from build123d import *

# Parameters (mm, degrees)
SKETCH1_W           = 114.24
SKETCH1_H           = 10
BOSS_EXTRUDE1_DEPTH = 10
SKETCH3_W           = 114.24
SKETCH3_H           = 10
BOSS_EXTRUDE2_DEPTH = 80
SKETCH4_R           = 4
CUT_EXTRUDE1_DEPTH  = 103.896522779


with BuildPart() as part:
    # Sketch1 → Boss-Extrude1 (new body)
    with BuildSketch(Plane.XY):
        Rectangle(SKETCH1_W, SKETCH1_H)
    extrude(amount=BOSS_EXTRUDE1_DEPTH)

    # Sketch3 → Boss-Extrude2 (add)
    with BuildSketch(Plane(origin=(0, 5, 0), x_dir=(1, 0, 0), z_dir=(0, 1, 0))):
        with Locations((0, -5)):
            Rectangle(SKETCH3_W, SKETCH3_H)
    extrude(amount=BOSS_EXTRUDE2_DEPTH)

    # Sketch4 → Cut-Extrude1 (cut, through all)
    with BuildSketch(Plane.XY.offset(10)):
        with Locations((24.87, 9.99)):
            Circle(SKETCH4_R)
    extrude(amount=-CUT_EXTRUDE1_DEPTH, mode=Mode.SUBTRACT)


solid = part.part
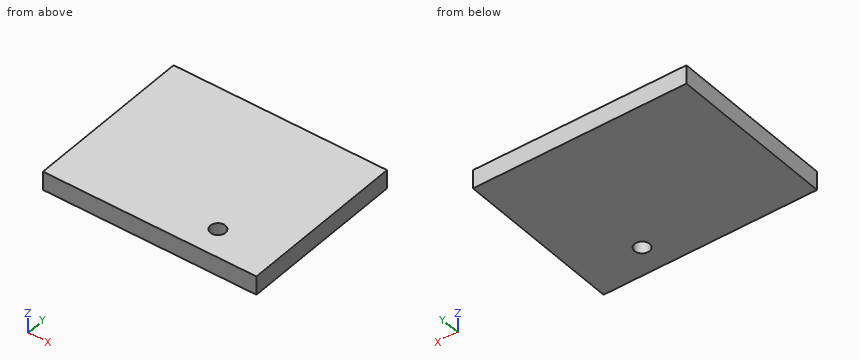
Here's how the part is built. I have some questions about the finished solid (model axes, mm). Round coordinates to 2 decimals unless told otherwise and drop trailing zeros. Write each loop counter-clockwise with the first axis right and the second up, starting at its lowest first coordinate (ties: lowest second). Pieces come first, ordered by that corner, then holes.
1. Suppose I cut it at A-A (y = 9.99). List the corners of the cut face in (x, z) for me.
2. Suppose I cut it at B-B (x = 24.87). List the corners of the cut face in (y, z) for me.
3. I need wall thicknesses on L1, parallel to Y at x = 24.87, z = 7.5; L2, parallel to X at y = 7, z = 0.5; L3, parallel to Y at x = 26, z = 9. Which ranges of each line are inside material? Lowest first, please.
Answer sheet:
1. outline: (-57.12, 0) - (20.87, 0) - (20.87, 10) - (-57.12, 10) - close; (28.87, 0) - (57.12, 0) - (57.12, 10) - (28.87, 10) - close
2. outline: (-5, 0) - (5.99, 0) - (5.99, 10) - (-5, 10) - close; (13.99, 0) - (85, 0) - (85, 10) - (13.99, 10) - close
3. L1: y = -5 to 5.99, 13.99 to 85
3. L2: x = -57.12 to 22.21, 27.53 to 57.12
3. L3: y = -5 to 6.15, 13.83 to 85
